from build123d import *

# Parameters (mm, degrees)
BOSS_EXTRUDE1_DEPTH = 108
BOSS_EXTRUDE3_REACH = 114.923
SKETCH5_W           = 13.804456559
SKETCH5_H           = 5
SKETCH7_W           = 12
SKETCH7_H           = 5
BOSS_EXTRUDE4_DEPTH = 9
SKETCH8_W           = 3.1
SKETCH8_H           = 5
CUT_EXTRUDE1_DEPTH  = 8
FILLET1_R           = 0.5
FILLET2_R           = 0.5
FILLET3_R           = 0.5
FILLET4_R           = 0.5
FILLET5_R           = 0.5
FILLET6_R           = 0.5
FILLET7_R           = 0.5
FILLET8_R           = 0.5
CUT_EXTRUDE2_DEPTH  = 10
FILLET9_R           = 3


with BuildPart() as part:
    # Sketch1 → Boss-Extrude1 (new body)
    with BuildSketch(Plane(origin=(0, 0, 0), x_dir=(0, 0, -1), z_dir=(1, 0, 0))):
        Polygon((32.5, -0.986763128), (32.5, -6.586763128), (30.340675248, -6.586763128), (30.340675248, -4.436763128), (28.831367778, -4.436763128), (28.831367778, -6.586763128), (-28.831367778, -6.586763128), (-28.831367778, -4.436763128), (-30.340675248, -4.436763128), (-30.340675248, -6.586763128), (-32.5, -6.586763128), (-32.5, -0.986763128), (-30.6, -0.986763128), (-30.6, -3.136763128), (-28.79, -3.136763128), (-28.79, -0.986763128), (28.79, -0.986763128), (28.79, -3.136763128), (30.6, -3.136763128), (30.6, -0.986763128), align=None)
    extrude(amount=BOSS_EXTRUDE1_DEPTH)

    # Sketch5 → Boss-Extrude3 (add, up to next)
    with BuildSketch(Plane(origin=(0, -0.986763128, 0), x_dir=(1, 0, 0), z_dir=(0, 1, 0)), mode=Mode.PRIVATE) as boss_extrude3_sk1:
        with Locations((101.097771721, -30)):
            Rectangle(SKETCH5_W, SKETCH5_H)
    boss_extrude3_tool1 = extrude(boss_extrude3_sk1.sketch, amount=-BOSS_EXTRUDE3_REACH, mode=Mode.PRIVATE) - part.part
    boss_extrude3 = boss_extrude3_tool1.solids().sort_by_distance((101.097772, -0.986763, 30))[0]
    add(boss_extrude3)

    # Sketch7 → Boss-Extrude4 (add)
    with BuildSketch(Plane(origin=(0, -0.986763128, 0), x_dir=(1, 0, 0), z_dir=(0, 1, 0))):
        with Locations((102, -30)):
            Rectangle(SKETCH7_W, SKETCH7_H)
    boss_extrude4 = extrude(amount=BOSS_EXTRUDE4_DEPTH)

    # Mirror1: Boss-Extrude4 across plane
    add(boss_extrude4.mirror(Plane.XY))

    # Mirror2: Boss-Extrude3 across plane
    add(boss_extrude3.mirror(Plane.XY))

    # Sketch8 → Cut-Extrude1 (cut)
    with BuildSketch(Plane(origin=(0, 8.013236872, 0), x_dir=(1, 0, 0), z_dir=(0, 1, 0))):
        with Locations((98.65, -30)):
            Rectangle(SKETCH8_W, SKETCH8_H)
    cut_extrude1 = extrude(amount=-CUT_EXTRUDE1_DEPTH, mode=Mode.SUBTRACT)

    # Mirror3: Cut-Extrude1 across plane
    add(cut_extrude1.mirror(Plane.XY), mode=Mode.SUBTRACT)

    # Fillet1
    fillet1_edges = [part.edges().sort_by_distance(p)[0] for p in [
        (47.09777172, -0.986763128, 30.6),
    ]]
    fillet(fillet1_edges, radius=FILLET1_R)

    # Fillet2
    fillet2_edges = [part.edges().sort_by_distance(p)[0] for p in [
        (47.09777172, -0.986763128, 28.79),
    ]]
    fillet(fillet2_edges, radius=FILLET2_R)

    # Fillet3
    fillet3_edges = [part.edges().sort_by_distance(p)[0] for p in [
        (54, -6.586763128, 30.340675248),
    ]]
    fillet(fillet3_edges, radius=FILLET3_R)

    # Fillet4
    fillet4_edges = [part.edges().sort_by_distance(p)[0] for p in [
        (54, -6.586763128, 28.831367778),
    ]]
    fillet(fillet4_edges, radius=FILLET4_R)

    # Fillet5
    fillet5_edges = [part.edges().sort_by_distance(p)[0] for p in [
        (104.1, 8.013236872, 32.5),
    ]]
    fillet(fillet5_edges, radius=FILLET5_R)

    # Fillet6
    fillet6_edges = [part.edges().sort_by_distance(p)[0] for p in [
        (96.55, 8.013236872, 32.5),
    ]]
    fillet(fillet6_edges, radius=FILLET6_R)

    # Fillet7
    fillet7_edges = [part.edges().sort_by_distance(p)[0] for p in [
        (47.09777172, -0.986763128, -28.79),
        (96.55, 8.013236872, 27.5),
        (104.1, 8.013236872, -32.5),
        (96.55, 8.013236872, -27.5),
        (54, -6.586763128, -32.5),
        (54, -6.586763128, -30.340675248),
        (54, -6.586763128, -28.831367778),
        (104.1, 8.013236872, 27.5),
        (96.55, 8.013236872, -32.5),
        (104.1, 8.013236872, -27.5),
    ]]
    fillet(fillet7_edges, radius=FILLET7_R)

    # Fillet8
    fillet8_edges = [part.edges().sort_by_distance(p)[0] for p in [
        (47.09777172, -0.986763128, -30.6),
    ]]
    fillet(fillet8_edges, radius=FILLET8_R)

    # Sketch9 → Cut-Extrude2 (cut)
    with BuildSketch(Plane(origin=(0, -0.986763128, 0), x_dir=(1, 0, 0), z_dir=(0, 1, 0))):
        with BuildLine():
            Line((90, -15), (90, 15))
            ThreePointArc((90, 15), (96, 21), (102, 15))
            Line((102, 15), (102, -15))
            ThreePointArc((102, -15), (96, -21), (90, -15))
        make_face()
        Polygon((86.8, 21.9), (79.3, 4.9), (12.3, 4.9), (4.8, 21.9), align=None)
        Polygon((4.8, -21.9), (86.8, -21.9), (79.3, -4.9), (12.3, -4.9), align=None)
    extrude(amount=-CUT_EXTRUDE2_DEPTH, mode=Mode.SUBTRACT)

    # Fillet9
    fillet9_edges = [part.edges().sort_by_distance(p)[0] for p in [
        (86.8, -3.786763128, 21.9),
        (4.8, -3.786763128, 21.9),
        (12.3, -3.786763128, 4.9),
        (79.3, -3.786763128, 4.9),
        (4.8, -3.786763128, -21.9),
        (86.8, -3.786763128, -21.9),
        (79.3, -3.786763128, -4.9),
        (12.3, -3.786763128, -4.9),
    ]]
    fillet(fillet9_edges, radius=FILLET9_R)


solid = part.part
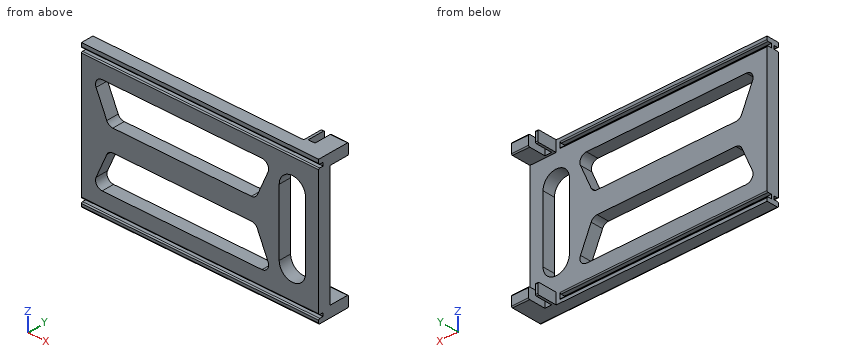
Verification items for the finished model (mm, model axes). Give positions to 0.01 mm unless a question says otherwise; leave off trailing zeros. Order: outer loops, then holes, each group sorted by start corner. A loop starts at its lowest first (then second) coordinate and runs counter-clockwise, first axis right, second up. Notation, with made-up numbers: M 66,40 L 102,40 A22 ccw 102,75 Z; hole C 58.25,13.5 d4. An arc over 180 degrees is marked long. Answer as a JSON object with one key per item and string values. Group by question number.
1) Depth check by flat-ended pin: pin 1 Ø0.6 at (y, z) = (-2.5, -29.5) entering from -X; pin 2 Ø4 at (y, z) = (3, 31) entering from -X; pin 3 Ø0.9 at (x, z) = (98, -31) entering from +Y. Enter the tip coordinate at first touch or a pass-through.
2) Scan lines: line 1 along Z through (x, y) = (5.5, -6); line 2 along Z through (x, y) = (27, -4.25); line 3 along Z through (x, y) = (96, -2). Record each from-to range of solid material in increasing order. Write a range as [from, to].
3) Cross-section at B-B (z = 8.5). Enter the section's corners in (x, y).
4) Cross-section at D-D (z = 24). Enter the section's corners in (x, y).
5) Cross-section at A-A (y = 6.25). Enter the section's corners in (x, z).
6) Cross-section at C-C (x = 63). Give the number of separate pieces and of enclosed holes in the cut face, then the cut area to 3 significant figures.
Result sheet:
{
 "1": {"pin 1": "stops at x = 94.2", "pin 2": "stops at x = 96", "pin 3": "stops at y = 0.01"},
 "2": {"line 1": "z = [-32.5, -30.34], [-28.83, 28.83], [30.34, 32.5]", "line 2": "z = [-32.5, -21.9], [-4.9, 4.9], [21.9, 32.5]", "line 3": "z = [-32.5, -21], [21, 32.5]"},
 "3": {"outline": "M 0,-6.59 L 10.71,-6.59 L 10.71,-0.99 L 0,-0.99 Z; M 80.89,-6.59 L 90,-6.59 L 90,-0.99 L 80.89,-0.99 Z; M 102,-6.59 L 108,-6.59 L 108,-0.99 L 102,-0.99 Z"},
 "4": {"outline": "M 0,-6.59 L 108,-6.59 L 108,-0.99 L 0,-0.99 Z"},
 "5": {"outline": "M 96,-32.5 L 97.1,-32.5 L 97.1,-27.5 L 96,-27.5 Z; M 96,27.5 L 97.1,27.5 L 97.1,32.5 L 96,32.5 Z; M 100.2,-32.5 L 108,-32.5 L 108,-27.5 L 100.2,-27.5 Z; M 100.2,27.5 L 108,27.5 L 108,32.5 L 100.2,32.5 Z"},
 "6": {"separate pieces": "3", "enclosed holes": "0", "area": "159 mm2"}
}
